Check sheet for the modelled part. Datum: model origin and axes. Units: mm. A direction names the side the tool comes from. Coordinates: 2 decimals unless noted, no trailing zeros. Write each loop counter-clockwise with the first axis right and the second up, starting at its lowest first coordinate (ties: lowest second). Pieces come first, ordered by that corner, then holes. Notation, with made-up numbers: M 55,30.25 L 107,30.25 A10 cw 107,44.25 Z; hole C 76,39 d4. An arc over 180 degrees is marked long. Answer as CSV lines item,"result". Start each with the question number.
1) Access from +Z, -Z, +X, -X, +Y, -Y to the whole of each face (thin tool, end or side, straight path). Record for faces 1 (the cylindrical face through (-0.54, -2.44, 4.93)), 2 (the flat face through (1.987, -0.226, 12.521)).
2) Draft check along X on faces 3 (the cylindrical face through (-1.08, -4.88, 10.49)), 4 (the flat face through (0, 0, 0)), 5 (the flat face through (-0.798, 1.834, 12.522)), 6 (the flat face through (-1.987, 0.226, 12.522)). Enter one of: +X half, -X half, draft (parallel to the pull), parting line (faces both ways), or undercut.
3) Material ranges on L1, parallel to Z at x = -1.25, y = -1.5; L2, parallel to X at y = 0, z = 13.5; L3, parallel to Y at x = 0, z = 3, recorded low to high. Write a range as [from, to].
4) Section check A-A (z = 4.5). Record the cut outline in (x, y).
5) Go/stop test with flat-tipped pins: pin 1 Ø1.5 at (x, z) = (1, 6.5) entering from -Y; pin 2 Ø2 at (x, z) = (-1.5, 4) entering from -Y; pin 3 Ø1.3 at (x, y) = (1, 0.5) entering from +Z. Record where each tip stops, or that it passes through.
from build123d import *

# Parameters (mm, degrees)
SKETCH_1_R          = 2.5
EXTRUDE_1_DEPTH     = 10
SKETCH_2_R          = 5
EXTRUDE_2_DEPTH     = 4
FILLET_1_R          = 3
CUT_EXTRUDE_1_DEPTH = 3


with BuildPart() as part:
    # 草图1 → 凸台-拉伸1 (new body)
    with BuildSketch(Plane.XY):
        Circle(SKETCH_1_R)
    extrude(amount=EXTRUDE_1_DEPTH)

    # 草图2 → 凸台-拉伸2 (add)
    with BuildSketch(Plane.XY.offset(10)):
        Circle(SKETCH_2_R)
    extrude(amount=EXTRUDE_2_DEPTH)

    # 圆角1
    fillet_1_edges = [part.edges().sort_by_distance(p)[0] for p in [
        (-5, 0, 14),
    ]]
    fillet(fillet_1_edges, radius=FILLET_1_R)

    # 草图3 → 切除-拉伸1 (cut)
    with BuildSketch(Plane.XY.offset(14)):
        Polygon((-0.242384409, -2.296646061), (1.867761628, -1.358234086), (2.110146037, 0.938411975), (0.242384409, 2.296646061), (-1.867761628, 1.358234086), (-2.110146037, -0.938411975), align=None)
    extrude(amount=-CUT_EXTRUDE_1_DEPTH, mode=Mode.SUBTRACT)


solid = part.part
Results found:
1,face 1,"-Z"
1,face 2,"+Z"
2,face 3,"parting line"
2,face 4,"draft"
2,face 5,"undercut"
2,face 6,"undercut"
3,L1,"z = [0, 11]"
3,L2,"x = [-3.66, -2.01], [2.01, 3.66]"
3,L3,"y = [-2.5, 2.5]"
4,outline,"C 0,0 d5"
5,pin 1,"stops at y = -2.49"
5,pin 2,"stops at y = -2.45"
5,pin 3,"stops at z = 11"
